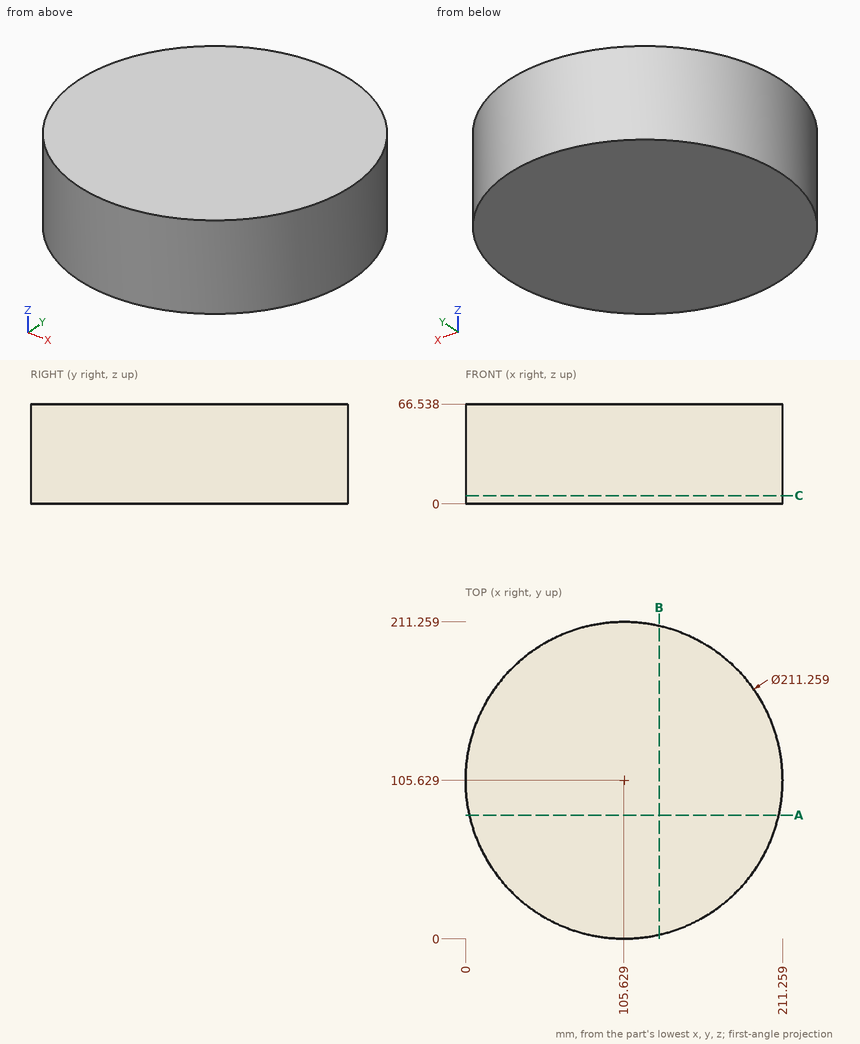
Verification items for this drawing (mm, ordinates from the low corner). Coordinates: 2 decimals unless noted, no trailing zeros. Loops run counter-clockwise (first coordinate to the right, second up) from the corner with the lowest first, then second, coordinate; pieces in that order, holes last. Notation, with made-up numbers: (-30, 69.25) - (-6, 69.25) arc R10 ccw to (-6, 78.25) - close; hole circle Ø4 at (60, 82). An arc over 180 degrees is marked (long way). Use one line per item in the form item = value. Start each with the question number.
Item 1: Gauge pin test, flat ends, axial feed: pin 1 (10 mm diameter, centred on x = 161, z = 20.5, fed in from +Y) (1 decimal); pin 2 (6 mm diameter, centred on y = 180, z = 7, fed in from +X); pin 3 (3 mm diameter, centred on y = 28, z = 7, fed in from +X) (1 decimal). Record the tip position at first contact, or that the pin passes through.
Item 2: Section check B-B, the plane x = 129. Enter the section's corners in (y, z), and give its area (3 significant figures).
Item 3: Section check C-C, the plane z = 5.5. Enter the section's corners in (x, y), and give its area (3 significant figures).
Item 4: Thickness scan on probe 1 along Y at (x, z) = (106, 64.5); probe 2 along Y at (x, z) = (168, 11.5); probe 3 along X at (y, z) = (160, 12.5). Record the ranges inside material, lowest first.
Item 5: Section check A-A, the plane y = 82.5. Enter the section's corners in (x, z) (1 decimal), and give its area (3 significant figures).
Computed:
q1.pin_1 = 198.5
q1.pin_2 = 183.5
q1.pin_3 = 178.9
q2.outline = (2.62, 0) - (208.64, 0) - (208.64, 66.54) - (2.62, 66.54) - close
q2.area = 13,700 mm2
q3.outline = circle Ø211.26 at (105.63, 105.63)
q3.area = 35,100 mm2
q4.probe_1 = 0 to 211.26
q4.probe_2 = 20.38 to 190.88
q4.probe_3 = 15.07 to 196.19
q5.outline = (2.6, 0) - (208.7, 0) - (208.7, 66.5) - (2.6, 66.5) - close
q5.area = 13,700 mm2
